Part model, mm, in its own coordinate system. Face numbers are marked on the shaded views. A direction names the side the tool comes from. Round coordinates to 2 decimals unless told otherwise and drop trailing zeros. Loops run counter-clockwise (first coordinate to the right, second up) from the corner with the lowest first, then second, coordinate; pieces in that order, holes last. Notation, with made-up numbers: M 37,30.25 L 72,30.25 A32 cw 72,62.25 Z; hole C 1,1 d3. An arc over 180 degrees is marked long. Put each result on its own line as item: value. Start each with the question number.
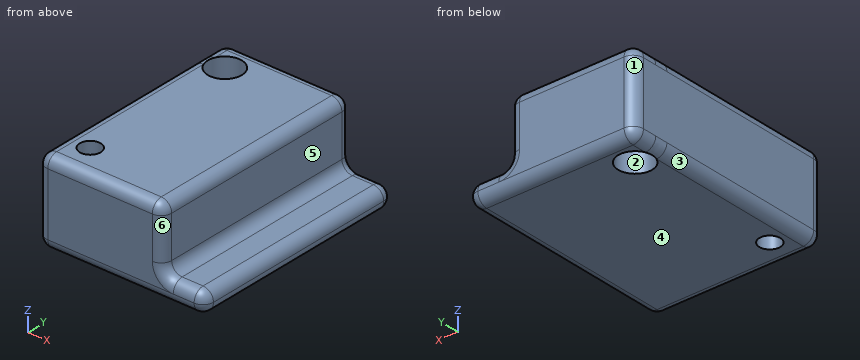
Autodesk Fusion 360 part; units mm, degrees
sketch "Main Body" plane through (0, 0, 0) normal (0, 0, 1) x (1, 0, 0)
  line L0 (0, 0) -> (16, 0)
  line L1 (16, 0) -> (16, 21.1)
  line L2 (16, 21.1) -> (0, 21.1)
  line L3 (0, 21.1) -> (0, 0)
  circle A0 centre (2.5, 18.1) radius 1.625
  line L4 (0, 10.55) -> (16, 10.55) construction
  circle A1 centre (2.5, 3) radius 1
  dimension "d1" = 16
  dimension "d2" = 21.1
  dimension "d3" = 3.25
  dimension "d4" = 3
  dimension "d5" = 2.5
  dimension "d6" = 10.55
  dimension "d11" = 2
  dimension "d12" = 2.5
  dimension "d13" = 3
extrude "Extrude1" add sketch "Main Body" along normal blind 8
sketch "step_cut" plane through (0, 0, 8) normal (0, 0, 1) x (-1, 0, 0)
  circle A0 centre (-2.5, -3) radius 1
  circle A1 centre (-2.5, -18.1) radius 1.625
  line L0 (0, -21.1) -> (0, 0)
  line L1 (0, 0) -> (-16, 0)
  line L2 (-16, 0) -> (-16, -21.1)
  line L3 (-16, -21.1) -> (0, -21.1)
  line L4 (-16, -21.1) -> (-12, -21.1)
  line L5 (-12, -21.1) -> (-12, 0)
  line L6 (-12, 0) -> (-16, 0)
  line L7 (-16, 0) -> (-16, -21.1)
extrude "Extrude2" cut sketch "step_cut" against normal blind 6 contours L1 L2 L3 L4 L5 L6 L7
fillet "Fillet1" radius 1 13 edges at (12, 10.55, 2) (12, 0, 5) (12, 21.1, 5) (0, 0, 4) (8, 0, 0) (16, 0, 1) (16, 21.1, 1) (16, 10.55, 0) (16, 10.55, 2) (14, 0, 2) (14, 21.1, 2) (12, 10.55, 8) (6, 0, 8) 2 faces at (0, 14.0667, 2.6667) (4, 21.1, 3.3333)
1. Which spindle directions (+Z, -Z, +X, -X, +Y, -Y) get a long thin tool onto all of the face, cutting with end or side? Do the marked faces 4, 5 and 6. Say none if no direction does.
2. Mould opens along Y. For the marked faces 1, 2 and 3 say: released by +Y, released by -Y, zero draft, split by the parting line, or undercut.
3. Drop flat-ended pins along their axis: pin 1 (3 mm diameter, centred on y = 17.5, z = 3, fed in from +X); pin 2 (1.2 mm diameter, centred on x = 2.5, y = 3, fed in from -Z); pin 3 (1.2 mm diameter, centred on y = 7, z = 4, fed in from +X); pin 4 (0.6 mm diameter, centred on x = 14, y = 7.5, fed in from +Z). Give the stop position or say it passes through.
4. Cut at C-C, the plane z = 4. Give the cut face in (x, y) (3 decimals), and give its area (3 significant figures).
5. Cut at B-B, the plane x = 2.5. Give the cut face in (y, z) (3 decimals), and give its area (3 significant figures).
6. Wall check: L1, parallel to Y at x = 2.5, z = 3.5 (3 decimals); L2, parallel to X at y = 18.1, z = 4.75 (3 decimals); L3, parallel to Y at x = 1.75, z = 7. Give the ranges that are in metal, low to high.
Results list:
1. face 4: -Z, +X, -X, +Y, -Y
1. face 5: +Z, +X, +Y, -Y
1. face 6: +Z, +X, -Y
2. face 1: released by +Y
2. face 2: undercut
2. face 3: zero draft
3. pin 1: stops at x = 15.87
3. pin 2: passes through
3. pin 3: stops at x = 12
3. pin 4: stops at z = 2
4. outline: M 0,1 A1 ccw 1,0 L 11,0 A1 ccw 12,1 L 12,20.1 A1 ccw 11,21.1 L 1,21.1 A1 ccw 0,20.1 Z; hole C 2.5,18.1 d3.25; hole C 2.5,3 d2
4. area: 241 mm^2
5. outline: M 0,1 A1 ccw 1,0 L 2,0 L 2,8 L 1,8 A1 ccw 0,7 Z; M 4,0 L 16.475,0 L 16.475,8 L 4,8 Z; M 19.725,0 L 20.1,0 A1 ccw 21.1,1 L 21.1,7 A1 ccw 20.1,8 L 19.725,8 Z
5. area: 126 mm^2
6. L1: y = 0 to 2, 4 to 16.475, 19.725 to 21.1
6. L2: x = 0 to 0.875, 4.125 to 12
6. L3: y = 0 to 2.34, 3.66 to 16.66, 19.54 to 21.1
